Could you check a few things on this model? Use its own coordinates, in mm. Give positions to 0.01 mm unless a question says otherwise; leave off trailing zeros. Order: outer loops, then holes, each group sorted by start corner. A loop starts at its lowest first (then second) coordinate and runs counter-clockwise, first axis right, second up. Notation, with made-up numbers: (30, 73) - (82, 73) arc R13 ccw to (82, 81) - close; hole circle Ø11 at (22.25, -2). An arc over 180 degrees is marked (long way). Put each result on its own line as item: value.
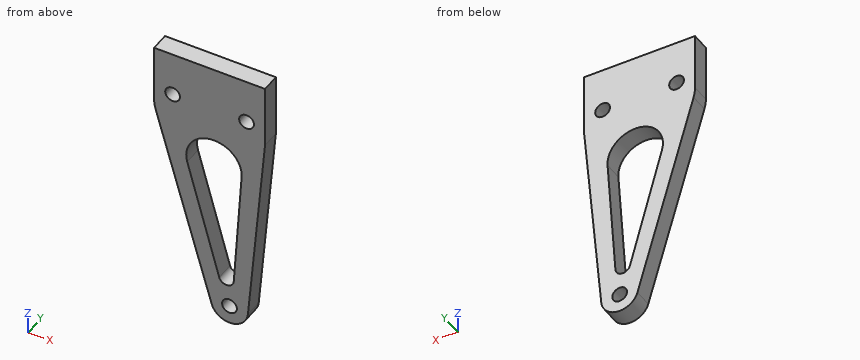
Autodesk Inventor part; units mm, degrees
ref_plane "YZ Plane" through (0, 0, 0) normal (1, 0, 0) x (0, 1, 0)
ref_plane "XZ Plane" through (0, 0, 0) normal (0, 1, 0) x (-1, 0, 0)
ref_plane "XY Plane" through (0, 0, 0) normal (0, 0, 1) x (1, 0, 0)
sketch "Boceto1" plane through (0, 0, 0) normal (1, 0, 0) x (0, 1, 0)
  point P0 (0, 0)
sketch "Boceto2" plane through (0, 0, 0) normal (0, 1, 0) x (-1, 0, 0)
  line L0 (0, 0) -> (30, 0)
  line L1 (30, 0) -> (30, -60)
  line L2 (30, -60) -> (0, -60)
  line L3 (0, -60) -> (0, 0)
  circle A0 centre (25, -5) radius 2
  line L4 (30, -30) -> (0, -30) construction
  circle A1 centre (25, -55) radius 2
  line L5 (15, 0) -> (15, -60) construction
  circle A2 centre (5, -5) radius 2
  circle A3 centre (5, -55) radius 2
  line L6 (0, -60) -> (4.6345, -112.9721)
  line L7 (0, -60) -> (53.1744, -60) construction
  line L8 (30, -60) -> (14.4189, -113.9242)
  line L9 (0, 0) -> (4.6345, 52.9721)
  line L10 (30, 0) -> (14.4189, 53.9242)
  arc A4 (14.4189, 53.9242) -> (4.6345, 52.9721) centre (9.6154, 52.5363) ccw
  arc A5 (4.6345, -112.9721) -> (14.4189, -113.9242) centre (9.6154, -112.5363) ccw
  circle A6 centre (9.6154, -112.5363) radius 2
  circle A7 centre (9.6154, 52.5363) radius 2
  line L11 (15, -60) -> (9.1311, -117.5128) construction
  line L12 (1.0267, -71.7351) -> (26.6092, -71.7351) construction
  arc A8 (21.0465, -73.7346) -> (6.3341, -72.2264) centre (13.818, -71.7351) ccw
  arc A9 (8.462, -104.6439) -> (12.3853, -105.0461) centre (10.4577, -104.5129) ccw
  line L13 (21.0465, -73.7346) -> (12.3853, -105.0461)
  line L14 (6.3018, -71.7351) -> (8.462, -104.6439)
  arc A10 (6.3341, 12.2264) -> (21.0465, 13.7346) centre (13.818, 11.7351) ccw
  arc A11 (12.3853, 45.0461) -> (8.462, 44.6439) centre (10.4577, 44.5129) ccw
  line L15 (21.0465, 13.7346) -> (12.3853, 45.0461)
  line L16 (6.3018, 11.7351) -> (8.462, 44.6439)
  point P0 (6.9725, -139.6956)
  point P1 (6.9725, 79.6956)
  dimension "d0" = 30
  dimension "d1" = 60
  dimension "d2" = 4
  dimension "d4" = 5
  dimension "d5" = 5
  dimension "d6" = 80
  dimension "d7" = 85
  dimension "d8" = 5
  dimension "d9" = 4
  dimension "d10" = 4
  dimension "d11" = 15
  dimension "d12" = 4
  dimension "d13" = 0.654
extrude "Extrusión1" add sketch "Boceto2" along normal blind 5
sketch "Boceto3" plane through (0, 5, 0) normal (0, 1, 0) x (1, 0, 0)
  point P0 (0, 0)
fillet "Empalme1" radius 10 2 edges at (-30, 2.5, 0) (-30, 2.5, -60)
sketch "Boceto5" plane through (0, 5, 0) normal (0, 1, 0) x (1, 0, 0)
  circle A0 centre (-5, 55) radius 2 construction
  line L0 (-5, 53) -> (-5, 43) construction
  line L1 (6.8466, 43) -> (-33.4625, 43)
  line L2 (-33.4625, 43) -> (-33.4625, -74.7352)
  line L3 (-33.4625, -74.7352) -> (6.8466, -74.7352)
  line L4 (6.8466, -74.7352) -> (6.8466, 43)
  point P0 (0, 0)
  dimension "d18" = 10
extrude "Extrusión2" cut sketch "Boceto5" against normal blind 10
1) Suppose I cut it at B-B, the plane z = -68. List the corners of the cut face in (x, y) for me.
Filled in:
outline: (-27.69, 0) - (-20.32, 0) - (-20.32, 5) - (-27.69, 5) - close; (-7.31, 0) - (-0.7, 0) - (-0.7, 5) - (-7.31, 5) - close
2) Suppose I cut it at C-C, the plane x = -25. List the corners of the cut face in (y, z) for me.
Filled in:
outline: (0, -77.3) - (5, -77.3) - (5, -57) - (0, -57) - close; (0, -53) - (5, -53) - (5, -43) - (0, -43) - close
3) Suppose I cut it at D-D, the plane y = 1.75. List the corners of the cut face in (x, z) for me, and give its area (3 significant figures).
Filled in:
outline: (-30, -58.58) arc R10 ccw to (-29.61, -61.36) - (-14.42, -113.92) arc R5 ccw to (-4.63, -112.97) - (0, -60) - (0, -43) - (-30, -43) - close; hole circle Ø4 at (-25, -55); hole (-21.05, -73.73) - (-12.39, -105.05) arc R2 ccw to (-8.46, -104.64) - (-6.33, -72.23) arc R7.5 ccw (long way) to start; hole circle Ø4 at (-9.62, -112.54); hole circle Ø4 at (-5, -55)
area: 1,160 mm^2
4) Suppose I cut it at A-A, the plane z = -55. List the corners of the cut face in (x, y) for me, and give its area (3 significant figures).
Filled in:
outline: (-30, 0) - (-27, 0) - (-27, 5) - (-30, 5) - close; (-23, 0) - (-7, 0) - (-7, 5) - (-23, 5) - close; (-3, 0) - (0, 0) - (0, 5) - (-3, 5) - close
area: 110 mm^2
5) I'm going to push flat-ended pins straight in: pin 1 (1 mm diameter, centred on y = 3.5, z = -95, fed in from +X); pin 2 (3 mm diameter, centred on y = 1.5, z = -101, fed in from +X); pin 3 (2 mm diameter, centred on y = 2.5, z = -62, fed in from +X); pin 4 (3.5 mm diameter, centred on x = -25, z = -55, fed in from -Y). Where does each tip first touch, or does it pass through?
Filled in:
pin 1: stops at x = -3.02
pin 2: stops at x = -3.46
pin 3: stops at x = -0.09
pin 4: passes through
6) If I drill on line 1 (X direction, y = 1.95, z = -54); line 2 (X direction, y = 2.85, z = -94.5); line 3 (X direction, y = 2.3, z = -93.5), over which ranges is the centre line in solid material (lowest first)? Write a range as [from, to].
Filled in:
line 1: x = [-30, -26.73], [-23.27, -6.73], [-3.27, 0]
line 2: x = [-20.03, -15.3], [-7.8, -3.02]
line 3: x = [-20.32, -15.58], [-7.73, -2.93]
